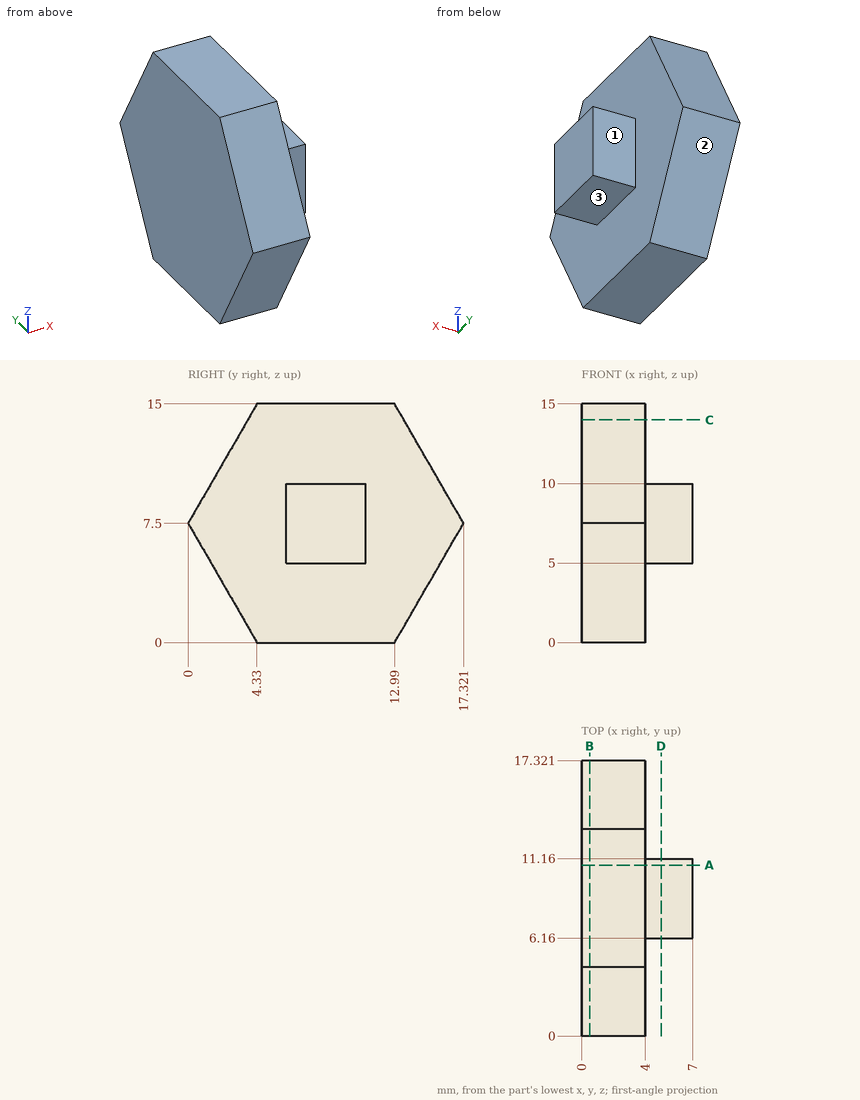
The drawing under review shows one solid part. Ordinate dimensions are in mm from its lowest x, y, z. A direction names the side the tool comes from. Round coordinates to 2 decimals unless told otherwise and drop trailing zeros. Loops run counter-clockwise (first coordinate to the right, second up) from the corner with the lowest first, then second, coordinate; pieces in that order, holes last. Notation, with made-up numbers: (-8, 8) - (38, 8) arc R20 ccw to (38, 14) - close; hole circle Ø11 at (-9.5, 29.5). An arc over 180 degrees is marked (long way). One line per question, with ' | ' between items.
1. For L1, parallel to X at y = 7.75, z = 14.5; L2, parallel to Z at x = 5, y = 10.25; L3, parallel to Z at x = 1.25, y = 2.25 (1 decimal), list the stretches that pass through material, from the lowest coordinate up. Write a range as [from, to].
Results are:
L1: x = [0, 4] | L2: z = [5, 10] | L3: z = [3.6, 11.4]
2. We need section C-C, the plane z = 14. State the section outline as (x, y) points.
Results are:
outline: (0, 3.75) - (4, 3.75) - (4, 13.57) - (0, 13.57) - close
3. For the marked faces 1, 2 and 3, list the 3-axis set-ups (+Z, -Z, +X, -X, +Y, -Y) from which the entire face can be reached by the end or side of a thin tool; tool diameter is ignored.
Results are:
face 1: +Z, -Z, +X, +Y | face 2: -Z, +X, -X, +Y | face 3: -Z, +X, +Y, -Y
4. We need section B-B, the plane x = 0.5. State the section outline as (y, z) points, and give its area (3 significant figures).
Results are:
outline: (0, 7.5) - (4.33, 0) - (12.99, 0) - (17.32, 7.5) - (12.99, 15) - (4.33, 15) - close | area: 195 mm²
5. We need section D-D, the plane x = 5. State the section outline as (y, z) points.
Results are:
outline: (6.16, 5) - (11.16, 5) - (11.16, 10) - (6.16, 10) - close
6. Clearance check with flat-ended pins moving along their axes: P1, Ø0.9, axis at x = 5.5, z = 7.5, coming from the -Y side; P2, Ø2.5, axis at x = 6, z = 8, coming from the +Y side; P3, Ø4, axis at y = 14, z = 7.5, coming from the +X side. State where each tip first meets the part, or that it passes through.
Results are:
P1: stops at y = 6.16 | P2: stops at y = 11.16 | P3: stops at x = 4
7. We need section A-A, the plane y = 10.75. State the section outline as (x, z) points.
Results are:
outline: (0, 0) - (4, 0) - (4, 5) - (7, 5) - (7, 10) - (4, 10) - (4, 15) - (0, 15) - close
